Solid Edge part; units mm, degrees
sketch "Sketch1" plane through (0, 0, 0) normal (0, 0, 1) x (1, 0, 0)
  line L0 (-26, -40) -> (26, -40)
  line L1 (26, -40) -> (26, 40)
  line L2 (26, 40) -> (-26, 40)
  line L3 (-26, 40) -> (-26, -40)
extrude "Protrusion1" add sketch "Sketch1" along normal blind 3
sketch "Sketch2" plane through (0, 0, 3) normal (0, 0, 1) x (-1, 0, 0)
  line L0 (-23, 14.4215) -> (-23, -40)
  line L1 (-23, -40) -> (-21.5, -40)
  line L2 (-21.5, -40) -> (-21.5, 12.9215)
  line L3 (-21.5, 12.9215) -> (-2.5, 12.9215)
  line L4 (-2.5, 12.9215) -> (-2.5, -0.5785)
  line L5 (-2.5, -0.5785) -> (-1, -0.5785)
  line L6 (-1, -0.5785) -> (-1, 14.4215)
  line L7 (-1, 14.4215) -> (-23, 14.4215)
  line L8 (-2.5, -40) -> (-1, -40)
  line L9 (-1, -40) -> (-1, -20)
  line L10 (-1, -20) -> (-2.5, -20)
  line L11 (-2.5, -20) -> (-2.5, -40)
extrude "ExtrudedProtrusion_2" add sketch "Sketch2" along normal blind 16.7
sketch "Sketch3" plane through (0, 0, 3) normal (0, 0, 1) x (-1, 0, 0)
  circle A0 centre (-7.15, 8.2) radius 1.5
  circle A1 centre (-16.6516, 8.2) radius 1.5011
extrude "Cutout1" cut sketch "Sketch3" against normal up to vertex (3 mm away)
sketch "Sketch4" plane through (0, 0, 3) normal (0, 0, 1) x (-1, 0, 0)
  circle A0 centre (2.2, 17.2) radius 1.5
  circle A1 centre (21, 33.2) radius 1.5
extrude "Cutout2" cut sketch "Sketch4" against normal up to vertex (3 mm away)
sketch "Sketch5" plane through (0, 0, 0) normal (0, 0, -1) x (-1, 0, 0)
  line L0 (33.5, 25) -> (26, 25)
  line L1 (26, 25) -> (26, 32.5)
  line L2 (26, 32.5) -> (33.5, 32.5)
  line L3 (33.5, 32.5) -> (33.5, 25)
  line L4 (33.5, -25) -> (26, -25)
  line L5 (26, -25) -> (26, -32.5)
  line L6 (26, -32.5) -> (33.5, -32.5)
  line L7 (33.5, -32.5) -> (33.5, -25)
  line L8 (-33.5, -25) -> (-26, -25)
  line L9 (-26, -25) -> (-26, -32.5)
  line L10 (-26, -32.5) -> (-33.5, -32.5)
  line L11 (-33.5, -32.5) -> (-33.5, -25)
  line L12 (-33.5, 25) -> (-26, 25)
  line L13 (-26, 25) -> (-26, 32.5)
  line L14 (-26, 32.5) -> (-33.5, 32.5)
  line L15 (-33.5, 32.5) -> (-33.5, 25)
extrude "Protrusion2" add sketch "Sketch5" against normal up to vertex (3 mm away)
sketch "Sketch6" plane through (0, 0, 3) normal (0, 0, 1) x (-1, 0, 0)
  line L0 (32, 25) -> (32, 32.5)
  line L1 (32, 32.5) -> (33.5, 32.5)
  line L2 (33.5, 32.5) -> (33.5, 25)
  line L3 (33.5, 25) -> (32, 25)
  line L4 (33.5, -32.5) -> (33.5, -25)
  line L5 (33.5, -25) -> (32, -25)
  line L6 (32, -25) -> (32, -32.5)
  line L7 (32, -32.5) -> (33.5, -32.5)
  line L8 (-32, -25) -> (-32, -32.5)
  line L9 (-32, -32.5) -> (-33.5, -32.5)
  line L10 (-33.5, -32.5) -> (-33.5, -25)
  line L11 (-33.5, -25) -> (-32, -25)
  line L12 (-33.5, 32.5) -> (-33.5, 25)
  line L13 (-33.5, 25) -> (-32, 25)
  line L14 (-32, 25) -> (-32, 32.5)
  line L15 (-32, 32.5) -> (-33.5, 32.5)
extrude "ExtrudedProtrusion_4" add sketch "Sketch6" along normal blind 1.5
sketch "Sketch7" plane through (0, 0, 0) normal (0, 0, -1) x (0, -1, 0)
  circle A0 centre (-25, 13) radius 7.5
  circle A1 centre (25, -13) radius 7.5
  circle A2 centre (-25, -13) radius 7.5
  circle A3 centre (25, 13) radius 7.5
extrude "Cutout3" cut sketch "Sketch7" against normal up to vertex (3 mm away)
fillet "Round_1" radius 3 4 edges at (1, -14.4215, 11.35) (2.5, -12.9215, 11.35) (21.5, -12.9215, 11.35) (23, -14.4215, 11.35)
fillet "Round_2" radius 1.35 6 edges at (1, -5.4215, 3) (1.8787, -13.5428, 3) (12, -14.4215, 3) (22.1213, -13.5428, 3) (23, 14.2893, 3) (1, 30, 3)
fillet "Round_3" radius 0.75 23 edges at (1, 40, 12.025) (0.6046, 40, 3.3954) (-13.175, 40, 3) (2.5, 40, 11.35) (-26, 0, 3) (-26, 36.25, 3) (-26, -36.25, 3) (0, -40, 3) (21.5, 40, 11.35) (23, 40, 12.025) (23.3954, 40, 3.3954) (25.175, 40, 3) (26, 36.25, 3) (26, 0, 3) (26, -36.25, 3) (-29, 32.5, 3) (-29, 25, 3) (-29, -25, 3) (-29, -32.5, 3) (29, 32.5, 3) (29, 25, 3) (29, -25, 3) (29, -32.5, 3)
sketch "Sketch8" plane through (0, 0.375, 3) normal (0, 0, 1) x (-1, 0, 0)
  circle A0 centre (0.7114, -8.8906) radius 2.3812
extrude "ExtrudedCutout_5" cut sketch "Sketch8" against normal blind 9.1795
properties material "ABS Plastic, medium impact"
Here's how the part is built. I have some questions about the finished solid (model axes, mm). A direction names the side the tool comes from. Give positions to 0.01 mm unless a question says otherwise; leave off trailing zeros. Loops run counter-clockwise (first coordinate to the right, second up) from the corner with the lowest first, then second, coordinate; pieces in that order, holes last. Notation, with made-up numbers: M -23.5,59 L 24.5,59 A7 ccw 24.5,71 Z; hole C -5,-4 d8. An arc over 180 degrees is marked long. Return JSON: item names as keys, results as strings.
Item 1: Imagine slicing it at B-B on x = -13. List the corners of the cut face in (y, z) for me, then the cut area to 3 significant figures.
A:
{"outline": "M -40,0 L -32.5,0 L -32.5,3 L -39.25,3 A0.75 ccw -40,2.25 Z; M -17.5,0 L 17.5,0 L 17.5,3 L -17.5,3 Z; M 32.5,0 L 40,0 L 40,2.25 A0.75 ccw 39.25,3 L 32.5,3 Z", "area": "150 mm^2"}
Item 2: Thinking about a two-plate mould opening in Y: for faces 1 (the flat face through (26, -36, 1)), 2 (the cylindrical face through (3.355, -12.019, 11.467)), 3 (the cylindrical face through (-0.401, 6.905, 1.521)), which applies, released by +Y, released by -Y, zero draft, split by the parting line, or undercut?
A:
{"face 1": "zero draft", "face 2": "released by +Y", "face 3": "undercut"}
Item 3: I'm going to push flat-ended pins straight in: pin 1 Ø2.5 at (y, z) = (-10.5, 1) entering from +X; pin 2 Ø3.5 at (y, z) = (-7.5, 11) entering from -X; pin 3 Ø10 at (y, z) = (-5.5, 4.5) entering from -X. Where does each tip first touch, or does it pass through?
A:
{"pin 1": "stops at x = 26", "pin 2": "stops at x = 1", "pin 3": "stops at x = -26"}
Item 4: Imagine slicing it at C-C on y = -8.2. List the corners of the cut face in (x, z) for me.
A:
{"outline": "M -26,0 L 5.65,0 L 5.65,3 L 2.5,3 L 2.5,19.7 L 1,19.7 L 1,4.35 A1.35 cw -0.35,3 L -25.25,3 A0.75 ccw -26,2.25 Z; M 8.65,0 L 15.15,0 L 15.15,3 L 8.65,3 Z; M 18.15,0 L 26,0 L 26,2.25 A0.75 ccw 25.25,3 L 24.35,3 A1.35 cw 23,4.35 L 23,19.7 L 21.5,19.7 L 21.5,3 L 18.15,3 Z"}
Item 5: On a 3-axis mill with a long thin cutter (end or side, diameter ignored), from which of +Z, -Z, +X, -X, +Y, -Y can I reach the whole of each face in a straight line? I mean faces 4 (the flat face through (2.5, 29, 11)), 5 (the flat face through (31, 25, 2)), 6 (the flat face through (-26, 36, 1)), 7 (the flat face through (-26, -36, 1)), 8 (the flat face through (1, -5, 12)). Say none if no direction works.
A:
{"face 4": "+Z, +Y", "face 5": "+Z, -Z, +X", "face 6": "+Z, -Z, -X, +Y", "face 7": "+Z, -Z, -X, -Y", "face 8": "+Z, -X, +Y, -Y"}
Item 6: Imagine slicing it at D-D on x = 6.5. List the corners of the cut face in (y, z) for me.
A:
{"outline": "M -40,0 L -28.74,0 L -28.74,3 L -39.25,3 A0.75 ccw -40,2.25 Z; M -21.26,0 L -9.55,0 L -9.55,3 L -12.92,3 L -12.92,19.7 L -14.42,19.7 L -14.42,4.35 A1.35 cw -15.77,3 L -21.26,3 Z; M -6.85,0 L 21.26,0 L 21.26,3 L -6.85,3 Z; M 28.74,0 L 40,0 L 40,3 L 28.74,3 Z"}
Item 7: Please list where these lines run through material, in increasing order: line 1 (X direction, y = -8.2, z = 1.55); line 2 (Y direction, x = 13, z = 0.9); line 3 (X direction, y = 36.5, z = 9.5).
A:
{"line 1": "x = -26 to 5.65, 8.65 to 15.15, 18.15 to 26", "line 2": "y = -40 to -32.5, -17.5 to 17.5, 32.5 to 40", "line 3": "x = 1 to 2.5, 21.5 to 23"}
